Autodesk Inventor part; units mm, degrees
ref_plane "XZ Plane" through (0, 0, 0) normal (0, 1, 0) x (-1, 0, 0)
ref_plane "XY Plane" through (0, 0, 0) normal (0, 0, 1) x (1, 0, 0)
sketch "Sketch1" plane through (0, 0, 0) normal (0, 1, 0) x (-1, 0, 0)
  line L0 (30.75, -15) -> (-30.75, -15)
  line L1 (-30.75, -15) -> (-30.75, 15)
  line L2 (-30.75, 15) -> (30.75, 15)
  line L3 (30.75, 15) -> (30.75, -15)
  point P0 (0, 0)
  point P1 (-30.75, 0)
  point P2 (0, -15)
  dimension "d0" = 61.5
  dimension "d1" = 30
extrude "Extrusion1" add sketch "Sketch1" along normal blind 2
sketch "Sketch2" plane through (30.75, 0, 15) normal (1, 0, 0) x (0, 0, -1)
  line L0 (0, 0) -> (30, 0) construction
  line L1 (0, 2) -> (30, 2) construction
  line L2 (0, 0) -> (0, 40)
  line L3 (30, 0) -> (30, 40)
  line L4 (0, 0) -> (30, 0)
  circle A0 centre (15, 35) radius 12 construction
  arc A1 (8.75, 35) -> (21.25, 35) centre (15, 35) ccw
  line L5 (8.75, 40) -> (8.75, 35)
  line L6 (21.25, 40) -> (21.25, 35)
  line L7 (0, 40) -> (8.75, 40)
  line L8 (21.25, 40) -> (30, 40)
  circle A2 centre (3, 35) radius 1.4
  circle A3 centre (6.5147, 26.5147) radius 1.4
  circle A4 centre (15, 23) radius 1.4
  circle A5 centre (23.4853, 26.5147) radius 1.4
  circle A6 centre (27, 35) radius 1.4
  point P0 (15, 0)
  point P1 (15, 2)
  point P2 (15, 28.75)
  dimension "d5" = 24
  dimension "d4" = 40
  dimension "d6" = 35
  dimension "d7" = 12.5
  dimension "d9" = 2.8
  dimension "d12" = 180
extrude "Extrusion2" add sketch "Sketch2" along normal blind 2
mirror "Mirror1" about plane through (0, 0, 0) normal (1, 0, 0) of "Extrusion2"
sketch "Sketch3" plane through (30.75, 2, 15) normal (0, 0, 1) x (1, 0, 0)
  line L0 (-63.5, 38) -> (-63.5, -2) construction
  line L1 (-63.5, 17.05) -> (-90.7062, -2)
  line L2 (-63.5, 17.05) -> (-63.5, -2)
  line L3 (-63.5, -2) -> (-90.7062, -2)
  point P0 (-30.75, -2)
  dimension "d16" = 19.05
  dimension "d17" = 55
extrude "Extrusion3" add sketch "Sketch3" against normal blind 30
mirror "Mirror2" about plane through (0, 0, 0) normal (1, 0, 0) of "Extrusion3"
sketch "Sketch4" plane through (0, 0, 0) normal (0, -1, 0) x (1, 0, 0)
  line L0 (-59.9562, 15) -> (59.9562, 15)
  line L1 (59.9562, 15) -> (59.9562, -15)
  line L2 (59.9562, -15) -> (-59.9562, -15)
  line L3 (-59.9562, -15) -> (-59.9562, 15)
  point P0 (0, 0)
extrude "Extrusion4" add sketch "Sketch4" along normal blind 25.4
sketch "Sketch5" plane through (0, -25.4, 0) normal (0, -1, 0) x (1, 0, 0)
  line L0 (-38.1, 38.1) -> (38.1, 38.1)
  line L1 (38.1, 38.1) -> (38.1, -38.1)
  line L2 (38.1, -38.1) -> (-38.1, -38.1)
  line L3 (-38.1, -38.1) -> (-38.1, 38.1)
  point P0 (0, 0)
  point P1 (0, 38.1)
  point P2 (38.1, 0)
  dimension "d22" = 76.2
  dimension "d23" = 76.2
extrude "Extrusion5" add sketch "Sketch5" along normal blind 228.6
sketch "Sketch6" plane through (30.75, 2, 15) normal (0, 0, 1) x (1, 0, 0)
  line L0 (-90.7062, -27.4) -> (-68.85, -58.6139)
  line L1 (-68.85, -27.4) -> (-68.85, -256) construction
  line L2 (-90.7062, -27.4) -> (-52.6011, -27.4) construction
  line L3 (-90.7062, -27.4) -> (-68.85, -27.4)
  line L4 (-68.85, -58.6139) -> (-68.85, -27.4)
  point P0 (-30.75, -2)
  dimension "d26" = 55
extrude "Extrusion6" add sketch "Sketch6" against normal blind 30
mirror "Mirror3" about plane through (0, 0, 0) normal (1, 0, 0) of "Extrusion6"
sketch "Sketch7" plane through (0, -254, 0) normal (0, -1, 0) x (1, 0, 0)
  line L0 (38.1, -38.1) -> (38.1, 38.1) construction
  line L1 (38.1, 38.1) -> (-38.1, 38.1) construction
  line L2 (25.4, -25.4) -> (-25.4, -25.4)
  line L3 (-25.4, -25.4) -> (-25.4, 25.4)
  line L4 (-25.4, 25.4) -> (25.4, 25.4)
  line L5 (25.4, 25.4) -> (25.4, -25.4)
  point P0 (0, 0)
  point P1 (0, 25.4)
  point P2 (0, 38.1)
  point P3 (25.4, 0)
  point P4 (38.1, 0)
  dimension "d29" = 50.8
  dimension "d30" = 50.8
extrude "Extrusion7" cut sketch "Sketch7" against normal blind 260.1875
properties part number "BiggerBracket"
Could you check a few things on this model? Use its own coordinates, in mm. A direction names the side the tool comes from. Coordinates: 2 decimals unless noted, no trailing zeros. Write each loop counter-clockwise with the first axis right and the second up, starting at its lowest first coordinate (ties: lowest second). Pieces come first, ordered by that corner, then holes. Notation, with made-up numbers: (89, 17.25) - (123, 17.25) arc R19 ccw to (123, 34.25) - close; hole circle Ø7 at (83.25, 18.25). An arc over 180 degrees is marked (long way). Put each result on its own line as item: value. Start each with the question number.
Q1. Please list where these lines run through material, in increasing order: L1, parallel to Z at x = 5, y = -40; L2, parallel to Y at x = 31.8, z = 0.
Q2. I want a section at C-C on y = -161.5. Write out the boundary of the cut face in (x, z).
Q3. I want a section at D-D on x = -50.5. Write out the boundary of the cut face in (y, z), plus the area to 3 significant figures.
Q4. I'm going to push flat-ended pins straight in: P1, Ø4.5, axis at x = 27.5, z = 2, coming from the +Y side; P2, Ø15, axis at y = -181.5, z = 3, coming from the -X side; P3, Ø4.5, axis at y = 26.51, z = -8.49, coming from the -X side; P4, Ø12, axis at x = 18, z = 14.5, coming from the +Y side. Where does each tip first touch, or does it pass through?
Q5. I want a section at A-A on x = 8. Write out the boundary of the cut face in (y, z), plus the area to 3 significant figures.
Q6. I want a section at B-B on y = -14.5. Write out the boundary of the cut face in (x, z).
Q7. Which directions (+Z, -Z, +X, -X, +Y, -Y) give clear straight access to the entire face, cutting with the end or side of a thin tool? Please do faces 4 (the flat face through (-1, -25.4, -29)), 5 (the flat face through (25.4, -128, 0)), 6 (the flat face through (32.75, 27, 0)).
Q8. Thinking about a two-plate mould opening in X: for faces 1 (the flat face through (-38.1, -138, -1)), 2 (the flat face through (0, -141, 25.4)), 3 (the flat face through (38.1, -138, 1)), which applies, pulls with the +X half, pulls with the -X half, needs draft (parallel to the pull), parting line crosses it, or undercut?
Checks:
1. L1: -38.1 to -25.4, 25.4 to 38.1
1. L2: -254 to 21.6, 24.4 to 28.75
2. outline: (-38.1, -38.1) - (38.1, -38.1) - (38.1, 38.1) - (-38.1, 38.1) - close; hole (-25.4, -25.4) - (25.4, -25.4) - (25.4, 25.4) - (-25.4, 25.4) - close
3. outline: (-38.9, -15) - (6.62, -15) - (6.62, 15) - (-38.9, 15) - close
3. area: 1,370 mm²
4. P1: y = 2
4. P2: x = -38.1
4. P3: x = -32.75
4. P4: through
5. outline: (-254, -38.1) - (-25.4, -38.1) - (-25.4, -25.4) - (-254, -25.4) - close; (-254, 25.4) - (-25.4, 25.4) - (-25.4, 38.1) - (-254, 38.1) - close
5. area: 5,810 mm²
6. outline: (-59.96, -15) - (-25.4, -15) - (-25.4, 15) - (-59.96, 15) - close; (25.4, -15) - (59.96, -15) - (59.96, 15) - (25.4, 15) - close
7. face 4: -Z, +X, -X, +Y
7. face 5: +Y, -Y
7. face 6: +Z, -Z, +X, +Y
8. face 1: pulls with the -X half
8. face 2: undercut
8. face 3: pulls with the +X half
